```python
from build123d import *

# Parameters (mm, degrees)
F0_R     = 3
F1_DEPTH = 1
F2_DEPTH = 10
F3_DEPTH = 9


with BuildPart() as f1:
    # F0 (on Top) → F1 (new body)
    with BuildSketch(Plane.XY):
        Polygon((5, -20), (5, 20), (-5, 20), (-5, -20), (0, -20), align=None)
        with BuildLine():
            ThreePointArc((3, -13.5), (2.12132, -15.62132), (0, -16.5))
            ThreePointArc((0, -16.5), (-3, -13.5), (0, -10.5))
            ThreePointArc((0, -10.5), (2.12132, -11.37868), (3, -13.5))
        make_face(mode=Mode.SUBTRACT)
        with BuildLine():
            ThreePointArc((3, -4.5), (2.12132, -6.62132), (0, -7.5))
            ThreePointArc((0, -7.5), (-2.12132, -2.37868), (3, -4.5))
        make_face(mode=Mode.SUBTRACT)
        with Locations((0, 4.5)):
            Circle(F0_R, mode=Mode.SUBTRACT)
        with Locations((0, 13.5)):
            Circle(F0_R, mode=Mode.SUBTRACT)
        Polygon((-5, 20), (5, 20), (5, -20), (0, -20), (-5, -20), (-5, -21), (6, -21), (6, 21), (-5, 21), align=None)
    extrude(amount=F1_DEPTH)

    # F0 (on Top) → F2 (join)
    with BuildSketch(Plane.XY):
        Polygon((-5, 23), (-5, 21), (6, 21), (6, -21), (-5, -21), (-5, -23), (8, -23), (8, 23), align=None)
    extrude(amount=F2_DEPTH)

    # F0 (on Top) → F3 (join)
    with BuildSketch(Plane.XY):
        with Locations((0, 13.5)):
            Circle(F0_R)
        with Locations((0, 4.5)):
            Circle(F0_R)
        with BuildLine():
            ThreePointArc((3, -4.5), (-2.12132, -2.37868), (0, -7.5))
            ThreePointArc((0, -7.5), (2.12132, -6.62132), (3, -4.5))
        make_face()
        with BuildLine():
            Line((0, -13.5), (0, -16.5))
            ThreePointArc((0, -16.5), (2.12132, -15.62132), (3, -13.5))
            ThreePointArc((3, -13.5), (2.12132, -11.37868), (0, -10.5))
            Line((0, -10.5), (0, -13.5))
        make_face()
        with BuildLine():
            ThreePointArc((0, -10.5), (-3, -13.5), (0, -16.5))
            Line((0, -16.5), (0, -13.5))
            Line((0, -13.5), (0, -10.5))
        make_face()
    extrude(amount=F3_DEPTH)


solid = f1.part
```
For this review, take the finished solid that the model builds, in its own axes (mm). A direction names the side the tool comes from. Coordinates: 2 decimals unless noted, no trailing zeros. Write each loop counter-clockwise with the first axis right and the second up, starting at its lowest first coordinate (ties: lowest second). Pieces come first, ordered by that corner, then holes. Notation, with made-up numbers: (-28.75, 29.25) -> (28.25, 29.25) arc R12 ccw to (28.25, 39.25) -> close; hole circle Ø11 at (9, 64). An arc over 180 degrees is marked (long way). Put each result on its own line as item: value.
Q1. The part is to be moulded in two halves that separate along Y. For faces 1 (the cylindrical face through (-0.65, 10.57, 4.94)), 2 (the flat face through (1, -23, 5)), 3 (the flat face through (8, 0, 5)), say which applies: +Y half, -Y half, draft (parallel to the pull), parting line (faces both ways), or undercut.
From the geometry:
face 1: undercut
face 2: -Y half
face 3: draft
Q2. Take a section at C-C, the plane x = 5.25. State the section outline as (y, z) points, then the cut area to 3 significant figures.
From the geometry:
outline: (-23, 0) -> (23, 0) -> (23, 10) -> (21, 10) -> (21, 1) -> (-21, 1) -> (-21, 10) -> (-23, 10) -> close
area: 82.0 mm2
Q3. Take a section at B-B, the plane z = 9.5. State the section outline as (x, y) points.
From the geometry:
outline: (-5, -23) -> (8, -23) -> (8, 23) -> (-5, 23) -> (-5, 21) -> (6, 21) -> (6, -21) -> (-5, -21) -> close
Q4. Tool access review of faces 4 (the flat face through (2, 23, 5)), 5 (the flat face through (0, -13, 9)), 6 (the flat face through (0, 0, 1)): name each direction out of +Z, -Z, +X, -X, +Y, -Y from which nothing blocks a thin tool from reaching the whole face with its end or side.
From the geometry:
face 4: +Z, -Z, +X, -X, +Y
face 5: +Z, -X
face 6: +Z
Q5. Take a section at A-A, the plane z = 2.75. State the section outline as (x, y) points, then the cut area to 3 significant figures.
From the geometry:
outline: (-5, -23) -> (8, -23) -> (8, 23) -> (-5, 23) -> (-5, 21) -> (6, 21) -> (6, -21) -> (-5, -21) -> close; circle Ø6 at (0, 4.5); circle Ø6 at (0, 13.5); (0, -16.5) arc R3 ccw to (3, -13.5) arc R3 ccw to (0, -10.5) arc R3 ccw to start; (0, -7.5) arc R3 ccw to (3, -4.5) arc R3 ccw (long way) to start
area: 249 mm2
Q6. Wall thickness on L1, parallel to Y at x = 2.25, z = 5; L2, parallel to Y at x = -1.5, z = 2.5; L3, parallel to Z at x = 3, y = -7.5: over which ranges is each line inside the solid? List them lowest first.
From the geometry:
L1: y = -23 to -21, -15.48 to -11.52, -6.48 to -2.52, 2.52 to 6.48, 11.52 to 15.48, 21 to 23
L2: y = -23 to -21, -16.1 to -10.9, -7.1 to -1.9, 1.9 to 7.1, 10.9 to 16.1, 21 to 23
L3: z = 0 to 1
Q7. Take a section at D-D, the plane y = 4.5. State the section outline as (x, z) points.
From the geometry:
outline: (-5, 0) -> (8, 0) -> (8, 10) -> (6, 10) -> (6, 1) -> (3, 1) -> (3, 9) -> (-3, 9) -> (-3, 1) -> (-5, 1) -> close
Q8. Clearance check with flat-ended pins moving along their axes: pin 1 Ø3 at (x, y) = (1.5, 3.5) entering from +Z; pin 2 Ø5 at (y, z) = (8.5, 6.5) entering from -X. State where each tip first meets the part, or that it passes through.
From the geometry:
pin 1: stops at z = 9
pin 2: stops at x = -2.6
